from build123d import *

# Parameters (mm, degrees)
BOSS_EXTRUDE1_DEPTH            = 3.175
HOLE_FOR_10_300_SC_NUTS_SP_1_D = 6.35


with BuildPart() as part:
    # Sketch1 → Boss-Extrude1 (new body)
    with BuildSketch(Plane(origin=(0, 0, 0), x_dir=(1, 0, 0), z_dir=(0, 1, 0))):
        with BuildLine():
            Line((-64.865326877, 53.014043584), (82.454673123, 53.014043584))
            ThreePointArc((82.454673123, 53.014043584), (84.250724348, 52.270094808), (84.994673123, 50.474043584))
            Line((84.994673123, 50.474043584), (84.994673123, -46.045956416))
            ThreePointArc((84.994673123, -46.045956416), (84.250724348, -47.842007641), (82.454673123, -48.585956416))
            Line((82.454673123, -48.585956416), (-64.865326877, -48.585956416))
            ThreePointArc((-64.865326877, -48.585956416), (-66.661378101, -47.842007641), (-67.405326877, -46.045956416))
            Line((-67.405326877, -46.045956416), (-67.405326877, 50.474043584))
            ThreePointArc((-67.405326877, 50.474043584), (-66.661378101, 52.270094808), (-64.865326877, 53.014043584))
        make_face()
    extrude(amount=BOSS_EXTRUDE1_DEPTH)

    # Hole for #10 300® SC Nuts (SP)1 (through all)
    with Locations(Plane(origin=(0, 0, 0), x_dir=(-1, 0, 0), z_dir=(0, -1, 0))):
        with Locations((-72.294673123, 46.664043584), (-72.294673123, -42.235956416), (54.705326877, -42.235956416), (54.705326877, 46.664043584)):
            Hole(HOLE_FOR_10_300_SC_NUTS_SP_1_D / 2)


solid = part.part
The listing builds one solid part. Answer for the finished solid, in the listing's coordinates (mm). Give positions to 0.01 mm unless a question says otherwise; leave off trailing zeros. Put each result on its own line as item: value.
Item 1: A straight line is drawn through the part: line 1 (X direction, y = 0.35, z = 43). Find the intervals that lie inside material, in ascending order.
Established:
line 1: x = -67.41 to -57.79, -51.62 to 69.21, 75.38 to 84.99
Item 2: For a pull along X with two mould halves and no side action, classify faces 1 (the face through (-53.24, 1.61, 45.053)), 2 (the face through (84.995, 2, -3)), 3 (the face through (10, 3.175, -3)) as released by +X, released by -X, zero draft, split by the parting line, or undercut.
Established:
face 1: undercut
face 2: released by +X
face 3: zero draft
Item 3: Given P1, Ø4, axis at x = -54.71, z = 42.24, coming from the +Y side, flat-ended and moving along its own axis, determine where the tip first touches the part or whether it passes through.
Established:
P1: passes through
